from build123d import *

# Parameters (mm, degrees)
F0_W     = 279.4
F0_H     = 508
F1_DEPTH = 19.05
F2_D     = 6.35
F3_D     = 6.35
F4_D     = 21.336


with BuildPart() as f1:
    # F0 (on Top) → F1 (new body)
    with BuildSketch(Plane.XY):
        with Locations((139.7, 254)):
            Rectangle(F0_W, F0_H)
    extrude(amount=F1_DEPTH)

    # F2 (through all)
    with Locations(Plane(origin=(0, 0, 0), x_dir=(1, 0, 0), z_dir=(0, 0, -1))):
        with Locations((19.05, -101.6), (260.35, -101.6), (260.35, -50.8), (19.05, -50.8)):
            Hole(F2_D / 2)

    # F3 (through all)
    with Locations(Plane(origin=(0, 0, 0), x_dir=(1, 0, 0), z_dir=(0, 0, -1))):
        with Locations((19.05, -441.325), (19.05, -422.275), (260.35, -422.275), (260.35, -441.325)):
            Hole(F3_D / 2)

    # F4 (through all)
    with Locations(Plane(origin=(0, 0, 0), x_dir=(1, 0, 0), z_dir=(0, 0, -1))):
        with Locations((38.1, -406.4), (241.3, -406.4), (139.7, -230.632)):
            Hole(F4_D / 2)


solid = f1.part
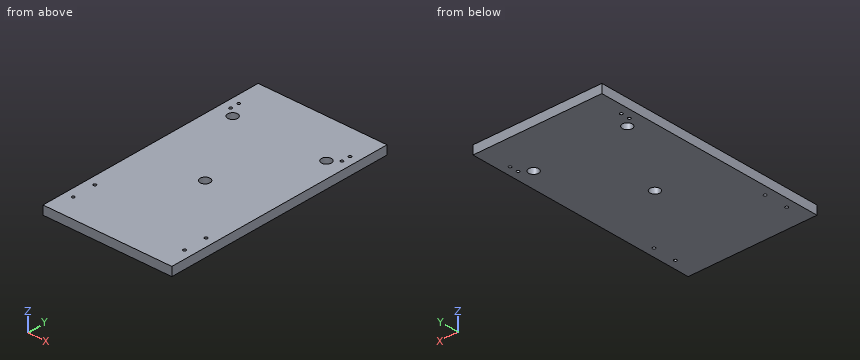
The model under review builds one solid part; all positions refer to its coordinate system, in mm. Give positions to 0.01 mm unless a question says otherwise; leave off trailing zeros. Loops run counter-clockwise (first coordinate to the right, second up) from the corner with the lowest first, then second, coordinate; pieces in that order, holes last. Notation, with made-up numbers: (-40, 6.25) -> (-22, 6.25) arc R19 cw to (-22, 10.25) -> close; hole circle Ø6 at (25.25, 1.5). An arc over 180 degrees is marked (long way). Put each result on its own line as item: value. Start each with the question number.
1. Wall thickness on probe 1 along Y at (x, z) = (19.05, 8) (3 decimals); probe 2 along X at (y, z) = (101.6, 4) (3 decimals); probe 3 along X at (y, z) = (406.4, 9): over which ranges is each line inside the solid? List them lowest first.
2. We need section A-A on x = 38.1. State the section outline as (y, z) points.
3. We need section B-B on y = 406.4. State the section outline as (x, z) points.
Determined:
1. probe 1: 0 to 47.625, 53.975 to 98.425, 104.775 to 419.1, 425.45 to 438.15, 444.5 to 508
1. probe 2: 0 to 15.875, 22.225 to 257.175, 263.525 to 279.4
1. probe 3: 0 to 27.43, 48.77 to 230.63, 251.97 to 279.4
2. outline: (0, 0) -> (395.73, 0) -> (395.73, 19.05) -> (0, 19.05) -> close; (417.07, 0) -> (508, 0) -> (508, 19.05) -> (417.07, 19.05) -> close
3. outline: (0, 0) -> (27.43, 0) -> (27.43, 19.05) -> (0, 19.05) -> close; (48.77, 0) -> (230.63, 0) -> (230.63, 19.05) -> (48.77, 19.05) -> close; (251.97, 0) -> (279.4, 0) -> (279.4, 19.05) -> (251.97, 19.05) -> close
